```python
from build123d import *

# Parameters (mm, degrees)
F1_DEPTH = 15
F4_DEPTH = 15


with BuildPart() as f1:
    # F0 (on Top) → F1 (new body)
    with BuildSketch(Plane.XY):
        Polygon((-15, 0), (0, 0), (0, -15), (15, -15), (15, 15), (-15, 15), align=None)
    extrude(amount=F1_DEPTH)

    # F3 (on offset) → F4 (join)
    with BuildSketch(Plane.XY.offset(14.8)):
        Polygon((14.851485, 0), (0, 0), (0, 15), (-15.148515, 15), (-15.148515, -15), (14.851485, -15), align=None)
    extrude(amount=F4_DEPTH)


solid = f1.part
```
The model under review builds one solid part; all positions refer to its coordinate system, in mm. A direction names the side the tool comes from. Round coordinates to 2 decimals unless told otherwise and drop trailing zeros. Write each loop counter-clockwise with the first axis right and the second up, starting at its lowest first coordinate (ties: lowest second). Pieces come first, ordered by that corner, then holes. Notation, with made-up numbers: (27, 44) - (45, 44) arc R23 ccw to (45, 71) - close; hole circle Ø1 at (82.25, 17.25). An arc over 180 degrees is marked (long way). One line per question, with ' | ' between items.
Item 1: Add section D-D, the plane y = -0.5. Give the boundary of the cut face in (x, z).
Resolved:
outline: (-15.15, 14.8) - (0, 14.8) - (0, 0) - (15, 0) - (15, 15) - (14.85, 15) - (14.85, 29.8) - (-15.15, 29.8) - close
Item 2: Add section A-A, the plane y = 7.75. Give the boundary of the cut face in (x, z), then the cut area to 3 significant figures.
Resolved:
outline: (-15.15, 14.8) - (-15, 14.8) - (-15, 0) - (15, 0) - (15, 15) - (0, 15) - (0, 29.8) - (-15.15, 29.8) - close | area: 674 mm2
Item 3: For P1, Ø7.5, axis at y = -4.5, z = 21.5, coming from the +X side; P2, Ø4.5, axis at x = 5, z = 25, coming from the +Y side, all flat-tipped, find the tip position at first contact; note any pin that passes through.
Resolved:
P1: stops at x = 14.85 | P2: stops at y = 0
Item 4: For faces 1 (the face through (14.851, -8, 22)), 2 (the face through (8, 0, 22)), 3 (the face through (-15, 8, 7)), 4 (the face through (-8, 0, 7)), list the 3-axis set-ups (+Z, -Z, +X, -X, +Y, -Y) from which the entire face can be reached by the end or side of a thin tool; tool diameter is ignored.
Resolved:
face 1: +Z, +X, +Y, -Y | face 2: +Z, +X, +Y | face 3: -Z, -X, +Y, -Y | face 4: -Z, -X, -Y
Item 5: To check wall thickness, follow probe 1 along Z at (x, y) = (12, 6.5); probe 2 along X at (y, z) = (7.5, 7.5); probe 3 along X at (y, z) = (2.25, 16.75). State the ranges of each line that lie inside material, in increasing order.
Resolved:
probe 1: z = 0 to 15 | probe 2: x = -15 to 15 | probe 3: x = -15.15 to 0
Item 6: Add section C-C, the plane x = 9. Give the boundary of the cut face in (y, z).
Resolved:
outline: (-15, 0) - (15, 0) - (15, 15) - (0, 15) - (0, 29.8) - (-15, 29.8) - close
Item 7: Add section B-B, the plane z = 10. Give the boundary of the cut face in (x, y), then the cut area to 3 significant figures.
Resolved:
outline: (-15, 0) - (0, 0) - (0, -15) - (15, -15) - (15, 15) - (-15, 15) - close | area: 675 mm2
